Work out the finished part from the listing and answer in its coordinate system (mm). A direction names the side the tool comes from. Give positions to 0.01 mm unless a question says otherwise; leave off trailing zeros. Loops run counter-clockwise (first coordinate to the right, second up) from the corner with the lowest first, then second, coordinate; pieces in that order, holes last. Notation, with made-up numbers: M 26,81.25 L 54,81.25 A22 cw 54,112.25 Z; hole C 21.5,8 d2. An arc over 180 degrees is marked long. Write item = value, one per line. Start each with the question number.
1. Consider L1, parallel to X at y = 15.75, z = -4; L2, parallel to Y at x = 22, z = -10; L3, parallel to X at y = 9, z = -23. Determine where each line is inside the solid, lowest interval first. Write a range as [from, to].
2. Flat-ended cylindrical pins translate along their axes: pin 1 Ø2 at (x, z) = (14, -43.5) entering from -Y; pin 2 Ø1 at (x, z) = (17, -9.5) entering from +Y; pin 3 Ø5.5 at (y, z) = (15, -7) entering from -X; pin 4 Ø6 at (y, z) = (13, -23) entering from -X. Find the tip coordinate at first contact, or state that the pin passes through.
3. The mould has two halves that part along Z. Classify faces 1 (the face through (41.38, 18.43, -1.1)), 2 (the face through (9.25, 16, -6)), 3 (the face through (28, 12, -5)): released by +Z, released by -Z, zero draft, split by the parting line, or undercut.
4. Section C-C on y = 6.75 is taken. Determine the outline of the cut face in (x, z).
5. Section A-A on z = -4.5 is taken. Determine the outline of the cut face in (x, y), plus the area to 3 significant figures.
6. Section B-B on x = 54 is taken. Determine the outline of the cut face in (y, z).
7. Section D-D on x = 20.95 is taken. Determine the outline of the cut face in (y, z), plus the area to 3 significant figures.
8. For faces 4 (the face through (29, 16, -7)), 5 (the face through (25, 1, -6)), 6 (the face through (15.016, 13.972, -6.997)), 7 (the face through (25, 10, -0.5)), determine the directions among +Z, -Z, +X, -X, +Y, -Y from which every point of the face is accessible in a straight line to the end or side of a thin tool.
```python
from build123d import *

# Parameters (mm, degrees)
SKETCH1_W           = 50
SKETCH1_H           = 50
BOSS_EXTRUDE1_DEPTH = 1
SKETCH2_W           = 50
SKETCH2_H           = 37.5
BOSS_EXTRUDE2_DEPTH = 19
SKETCH3_W           = 34
SKETCH3_H           = 14
BOSS_EXTRUDE3_DEPTH = 12
SKETCH4_R           = 2
BOSS_EXTRUDE4_DEPTH = 1.5
SKETCH5_W           = 7
SKETCH5_H           = 12
CUT_EXTRUDE1_DEPTH  = 7
FILLET1_R           = 2
SKETCH6_R           = 2.32139267
BOSS_EXTRUDE5_DEPTH = 4
LPATTERN1_COUNT     = 4
LPATTERN1_PITCH     = 8.2


with BuildPart() as part:
    # Sketch1 → Boss-Extrude1 (new body)
    with BuildSketch(Plane(origin=(0, 0, 0), x_dir=(1, 0, 0), z_dir=(0, 1, 0))):
        with Locations((25, 25)):
            Rectangle(SKETCH1_W, SKETCH1_H)
    extrude(amount=BOSS_EXTRUDE1_DEPTH)

    # Sketch2 → Boss-Extrude2 (add)
    with BuildSketch(Plane(origin=(0, 1, 0), x_dir=(1, 0, 0), z_dir=(0, 1, 0))):
        with Locations((25, 31.25)):
            Rectangle(SKETCH2_W, SKETCH2_H)
    extrude(amount=BOSS_EXTRUDE2_DEPTH)

    # Sketch3 → Boss-Extrude3 (add)
    with BuildSketch(Plane.XY.offset(-12.5)):
        with Locations((25, 12)):
            Rectangle(SKETCH3_W, SKETCH3_H)
    extrude(amount=BOSS_EXTRUDE3_DEPTH)

    # Sketch4 → Boss-Extrude4 (add)
    with BuildSketch(Plane.XZ):
        with BuildLine():
            Line((0, -32.003753373), (-6.121503896, -37.739612135))
            ThreePointArc((-6.121503896, -37.739612135), (-7.102759148, -40.003753373), (-6.121503896, -42.267894612))
            Line((-6.121503896, -42.267894612), (0, -48.003753373))
            Line((0, -48.003753373), (0, -32.003753373))
        make_face()
        with Locations(Location((-4, -40.003753373, 0), (0, 0, 270))):
            Circle(SKETCH4_R, mode=Mode.SUBTRACT)
    boss_extrude4 = extrude(amount=-BOSS_EXTRUDE4_DEPTH)

    # Mirror1: Boss-Extrude4 across plane
    add(boss_extrude4.mirror(Plane.ZY.offset(-25)))

    # Sketch5 → Cut-Extrude1 (cut)
    with BuildSketch(Plane(origin=(0, 19, 0), x_dir=(1, 0, 0), z_dir=(0, 1, 0))):
        with Locations((21, 6.5)):
            Rectangle(SKETCH5_W, SKETCH5_H)
        with Locations((29, 6.5)):
            Rectangle(SKETCH5_W, SKETCH5_H)
        with Locations((37.25, 6.5)):
            Rectangle(SKETCH5_W, SKETCH5_H)
        with Locations((12.75, 6.5)):
            Rectangle(SKETCH5_W, SKETCH5_H)
    extrude(amount=-CUT_EXTRUDE1_DEPTH, mode=Mode.SUBTRACT)

    # Fillet1
    fillet1_edges = [part.edges().sort_by_distance(p)[0] for p in [
        (41.375, 19, -0.5),
        (33.125, 19, -0.5),
        (25, 19, -0.5),
        (16.875, 19, -0.5),
        (8.625, 19, -0.5),
    ]]
    fillet(fillet1_edges, radius=FILLET1_R)

    # Sketch6 → Boss-Extrude5 (add)
    with BuildSketch(Plane(origin=(0, 12, 0), x_dir=(1, 0, 0), z_dir=(0, 1, 0))):
        with Locations(Location((12.75, 7.5, 0), (0, 0, 90))):
            Circle(SKETCH6_R)
    boss_extrude5 = extrude(amount=BOSS_EXTRUDE5_DEPTH)

    # LPattern1: Boss-Extrude5 ×4
    with Locations(*[(i * LPATTERN1_PITCH, 0, 0) for i in range(1, LPATTERN1_COUNT)]):
        add(boss_extrude5)


solid = part.part
```
Verdict:
q1.L1 = [8, 9.25], [16.25, 17.5], [24.5, 25.5], [32.5, 33.75], [40.75, 42]
q1.L2 = [0, 1], [5, 12]
q1.L3 = [0, 50]
q2.pin_1 = 0
q2.pin_2 = 19
q2.pin_3 = 8
q2.pin_4 = 0
q3.face_1 = released by +Z
q3.face_2 = zero draft
q3.face_3 = undercut
q4.outline = M 0,-50 L 50,-50 L 50,-12.5 L 42,-12.5 L 42,-0.5 L 8,-0.5 L 8,-12.5 L 0,-12.5 Z
q5.outline = M 0,0 L 50,0 L 50,1 L 0,1 Z; M 8,5 L 42,5 L 42,19 L 40.75,19 L 40.75,12 L 33.75,12 L 33.75,19 L 32.5,19 L 32.5,12 L 25.5,12 L 25.5,19 L 24.5,19 L 24.5,12 L 17.5,12 L 17.5,19 L 16.25,19 L 16.25,12 L 9.25,12 L 9.25,19 L 8,19 Z
q5.area = 330 mm2
q6.outline = M 0,-44.26 L 1.5,-44.26 L 1.5,-42 L 0,-42 Z; M 0,-38 L 1.5,-38 L 1.5,-35.75 L 0,-35.75 Z
q7.outline = M 0,-50 L 20,-50 L 20,-12.5 L 12,-12.5 L 12,-9.82 L 16,-9.82 L 16,-5.18 L 12,-5.18 L 12,-0.5 L 5,-0.5 L 5,-12.5 L 1,-12.5 L 1,0 L 0,0 Z
q7.area = 865 mm2
q8.face_4 = +Z, +Y
q8.face_5 = +Z, +X, -X
q8.face_6 = +Y
q8.face_7 = +Z, +X, -X, +Y
